Can you work these out from the model? Positions are in its coordinate system, mm. Face numbers are marked on the shaded views. A direction names the side the tool comes from. Round coordinates to 2 decimals unless told otherwise and drop trailing zeros. Loops run counter-clockwise (first coordinate to the right, second up) from the corner with the lowest first, then second, coordinate; pieces in that order, holes last. Notation, with made-up numbers: M 39,61.25 L 59,61.25 A19 ccw 59,73.25 Z; hole C -23,63 d2. An arc over 180 degrees is marked long. Answer as CSV lines item,"result".
from build123d import *

# Parameters (mm, degrees)
F1_DEPTH = 88.9
F2_DEPTH = 38.1
F3_W     = 3.048
F3_H     = 6.096
F4_DEPTH = 76.201
F5_R     = 5.07999


# Not quite as in the source:
# - a fillet or chamfer is up to 0.001 mm smaller than in the source, because OpenCascade refuses the exact size


with BuildPart() as f1:
    # F0 (on Top) → F1 (new body)
    with BuildSketch(Plane.XY):
        Polygon((-3.5306826939, -16.4269548038), (-16.2306826939, -16.4269548038), (-38.1, -16.4269548038), (-38.1, -21.5069548038), (38.1, -21.5069548038), (38.1, -16.4269548038), (16.2306826939, -16.4269548038), (3.5306826939, -16.4269548038), align=None)
    extrude(amount=F1_DEPTH)

    # F0 (on Top) → F2 (join)
    with BuildSketch(Plane.XY):
        with BuildLine():
            ThreePointArc((14.265, 0), (0, -14.265), (-14.265, 0))
            Line((-14.265, 0), (-16.8021, 0))
            ThreePointArc((-16.8021, 0), (-16.6586331687, -2.1910055589), (-16.2306826939, -4.344594768))
            Line((-16.2306826939, -4.344594768), (-16.2306826939, -16.4269548038))
            Line((-16.2306826939, -16.4269548038), (-3.5306826939, -16.4269548038))
            Line((-3.5306826939, -16.4269548038), (3.5306826939, -16.4269548038))
            Line((3.5306826939, -16.4269548038), (16.2306826939, -16.4269548038))
            Line((16.2306826939, -16.4269548038), (16.2306826939, -4.344594768))
            ThreePointArc((16.2306826939, -4.344594768), (16.6586331687, -2.1910055589), (16.8021, 0))
            Line((16.8021, 0), (14.265, 0))
        make_face()
    extrude(amount=F2_DEPTH)

    # F3 (on face) → F4 (cut, through all)
    with BuildSketch(Plane.YZ.offset(38.1)):
        with Locations((-14.9029548038, 8.7181735593)):
            Rectangle(F3_W, F3_H)
        with Locations((-14.9029548038, 28.7483400475)):
            Rectangle(F3_W, F3_H)
    extrude(amount=-F4_DEPTH, mode=Mode.SUBTRACT)

    # F5 (radius 5.08 in the source; OpenCascade refuses exactly that, so slightly less here)
    f5_edges = [f1.edges().sort_by_distance(p)[0] for p in [
        (0, -16.426955, 88.9),
        (38.1, -16.426955, 44.45),
        (27.165341, -16.426955, 0),
        (-38.1, -16.426955, 44.45),
        (-27.165341, -16.426955, 0),
        (16.230683, -10.385775, 38.1),
        (-16.230683, -10.385775, 38.1),
    ]]
    fillet(f5_edges, radius=F5_R)


solid = f1.part
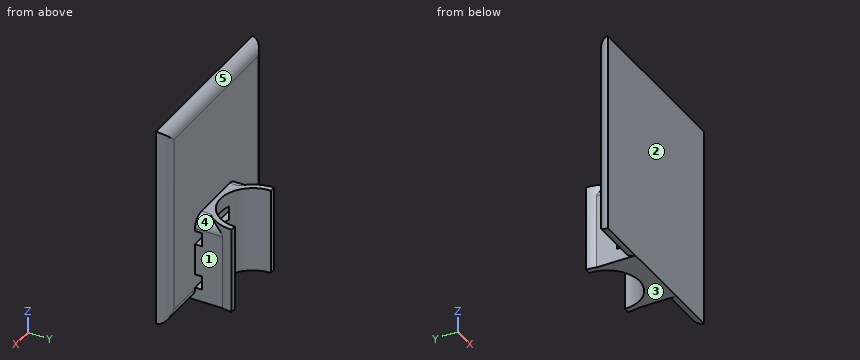
Item 1: On a 3-axis mill with a long thin cutter (end or side, diameter ignored), from which of +Z, -Z, +X, -X, +Y, -Y can I reach the whole of each face in a straight line? I mean the marked faces 4 and 5. Say none if no direction works.
Output:
face 4,"+Z, +X"
face 5,"+Z, +X, -X, +Y"
Item 2: If I drill on line 1 along Y through (x, z) = (30, 78); line 2 along Y through (x, z) = (-13, 11); line 3 along X through (y, z) = (-12.75, 33), over which ranges is the centre line in solid material (lowest first)? Write a range as from..to.
Output:
line 1,"y = -21.51..-16.43"
line 2,"y = -21.51..-16.43, -13.38..-5.87"
line 3,"x = -16.23..-6.4, 6.4..16.23"
Item 3: Will these pins go through, and if not, where does the flat tip stop? pin 1 (4 mm diameter, centred on y = -13, z = 73, fed in from -X); pin 2 (8.5 mm diameter, centred on y = -17, z = 24.5, fed in from +X); pin 3 (1.5 mm diameter, centred on x = 2.5, y = -15.5, fed in from +Z); pin 4 (20 mm diameter, centred on x = 2.5, z = 49.5, fed in from +Y).
Output:
pin 1,"passes through"
pin 2,"stops at x = 38.09"
pin 3,"stops at z = 38.1"
pin 4,"stops at y = -16.43"
Item 4: We'd pull the mould along Y, two halves only. Please class the marked faces 1, 2 and 3: released by +Y, released by -Y, zero draft, split by the parting line, or undercut.
Output:
face 1,"undercut"
face 2,"released by -Y"
face 3,"zero draft"
Item 5: If we section it at D-D on x = 13: State how many separate pieces and enclosed holes the cut face has, then the cut area to 3 significant figures.
Output:
separate pieces,"1"
enclosed holes,"2"
area,"809 mm2"
Item 6: If we section it at B-B on y = -6.75: Write out the boundary of the cut face in (x, z), then the cut area to 3 significant figures.
Output:
outline,"M -16.23,0 L -12.57,0 L -12.57,38.1 L -15.39,38.1 L -15.39,35.82 A5.08 ccw -16.23,33.02 Z; M 12.57,0 L 16.23,0 L 16.23,33.02 A5.08 ccw 15.39,35.82 L 15.39,38.1 L 12.57,38.1 Z"
area,"274 mm2"
